from build123d import *

# Parameters (mm, degrees)
BOSS_EXTRUDE1_DEPTH = 2.54
CUT_EXTRUDE2_DEPTH  = 2.032


with BuildPart() as part:
    # Sketch1 → Boss-Extrude1 (new body)
    with BuildSketch(Plane.XY):
        Polygon((-27.94, 0), (-10.16, 0), (-10.16, 5.08), (-6.368400563, 0), (-2.576801125, 5.08), (1.214798312, 0), (5.006397749, 5.08), (8.797997187, 0), (12.589596624, 5.08), (16.381196061, 0), (20.172795499, 5.08), (23.964394936, 0), (27.94, 5.08), (27.94, 10.16), (-27.94, 10.16), align=None)
    extrude(amount=BOSS_EXTRUDE1_DEPTH)

    # Sketch2 → Cut-Extrude2 (cut)
    with BuildSketch(Plane.XZ):
        with BuildLine():
            Line((-27.94, 0), (-13.275788511, 0))
            ThreePointArc((-13.275788511, 0), (-12.7, 1.27), (-13.275788511, 2.54))
            Line((-13.275788511, 2.54), (-27.94, 2.54))
            Line((-27.94, 2.54), (-27.94, 0))
        make_face()
    extrude(amount=-CUT_EXTRUDE2_DEPTH, mode=Mode.SUBTRACT)


solid = part.part
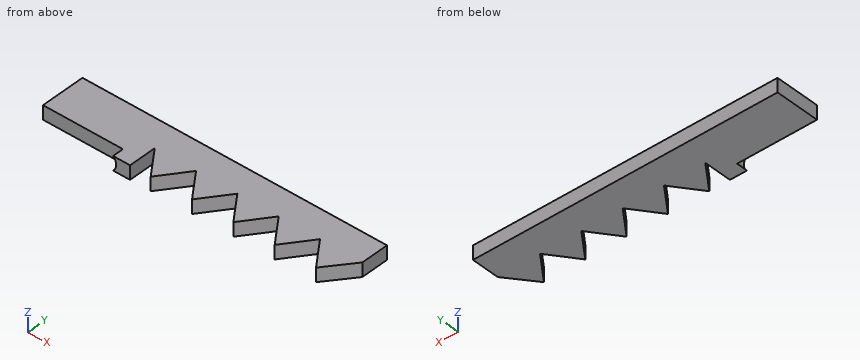
Can you work these out from the model? Positions are in its coordinate system, mm. Round coordinates to 2 decimals unless told otherwise and drop trailing zeros. Write each loop counter-clockwise with the first axis right and the second up, starting at its lowest first coordinate (ties: lowest second). Pieces come first, ordered by that corner, then holes. Notation, with made-up numbers: (30, 46.25) - (41, 46.25) arc R23 ccw to (41, 76.25) - close; hole circle Ø9 at (71.5, 70). An arc over 180 degrees is marked (long way). Write each question's results on one line, items separated by ' | '. Start each with the question number.
1) For pin 1 Ø1.5 at (y, z) = (1, 0.5) entering from +X; pin 2 Ø1 at (x, z) = (4.5, 1) entering from -Y, each with a flat end and sliding along its axis, tell me the tip position at first contact or that it passes through.
2) Please list where these lines run through material, in increasing order: line 1 (X direction, y = 2.5, z = 0.55); line 2 (X direction, y = 2, z = 0.2); line 3 (Y direction, x = -17.5, z = 1.45).
3) Suppose I cut it at B-B (x = 22). List the corners of the cut face in (y, z) for me.
4) Suppose I cut it at C-C (x = 0). List the corners of the cut face in (y, z) for me, and give its area (3 significant figures).
5) Suppose I cut it at A-A (z = 1.2). List the corners of the cut face in (x, y) for me.
Here are the results:
1) pin 1: stops at x = 25.33 | pin 2: stops at y = 3.73
2) line 1: x = -27.94 to -10.16, -8.23 to -4.5, -0.65 to 3.08, 6.93 to 10.66, 14.52 to 18.25, 22.1 to 25.92 | line 2: x = -13.08 to -10.16, -7.86 to -4.88, -0.28 to 2.71, 7.31 to 10.29, 14.89 to 17.87, 22.47 to 25.53 | line 3: y = 2.03 to 10.16
3) outline: (2.63, 0) - (10.16, 0) - (10.16, 2.54) - (2.63, 2.54) - close
4) outline: (1.63, 0) - (10.16, 0) - (10.16, 2.54) - (1.63, 2.54) - close | area: 21.7 mm2
5) outline: (-27.94, 2.03) - (-12.7, 2.03) - (-12.7, 0) - (-10.16, 0) - (-10.16, 5.08) - (-6.37, 0) - (-2.58, 5.08) - (1.21, 0) - (5.01, 5.08) - (8.8, 0) - (12.59, 5.08) - (16.38, 0) - (20.17, 5.08) - (23.96, 0) - (27.94, 5.08) - (27.94, 10.16) - (-27.94, 10.16) - close
